Design review of the part built by this model. Coordinates are the model's own, in mm. A direction names the side the tool comes from. Coordinates: 2 decimals unless noted, no trailing zeros. Loops run counter-clockwise (first coordinate to the right, second up) from the corner with the lowest first, then second, coordinate; pieces in that order, holes last.
Q1. Wall thickness on probe 1 along X at (y, z) = (-3.05, -19); probe 2 along Z at (x, y) = (1.5, 2.5); probe 3 along Z at (x, y) = (1.5, 0): over which ranges is each line inside the solid? List them lowest first.
Q2. Add section B-B on x = 3.5. Give the boundary of the cut face in (y, z), and give its area (3 significant figures).
Q3. For P1, Ø2, axis at x = 6.5, y = 0.5, coming from the -Z side; P2, Ø3.5, axis at x = 5, z = -19, coming from the +Y side; P3, Ø5, axis at x = 7.5, z = -13, coming from the +Y side; P4, Ø3, axis at x = 2.5, z = -17.5, coming from the +Y side, all flat-tipped, find the tip position at first contact; note any pin that passes through.
Q4. Draft analysis for pull direction Z (two halves, no side actions). For faces 6 (the face through (0, 2, 0)), 7 (the face through (5, 1, -11.5)), 8 (the face through (5, -4, -3.15)), state which applies: released by +Z, released by -Z, zero draft, split by the parting line, or undercut.
Q5. Machinability: for faces 1 (the face through (2.7, -1, -16.8)), 2 (the face through (5, -4, 3.15)), 3 (the face through (5, 1, 11.5)), 4 (the face through (3.2, -3, -21.4)), 5 (the face through (1, -3, -24)), which of the approach directions +Z, -Z, +X, -X, +Y, -Y give a long, thin tool a straight path to every point of the face, cutting with its end or side? Answer none if there is none.
Q6. Add section C-C on z = 16.5. Give the boundary of the cut face in (x, y), and give its area (3 significant figures).
Q7. Add section A-A on z = -19. Give the boundary of the cut face in (x, y).
Q8. Add section D-D on z = -12.5. Give the boundary of the cut face in (x, y).
```python
from build123d import *

# Parameters (mm, degrees)
SKETCH1_W           = 50
SKETCH1_H           = 10
BOSS_EXTRUDE1_DEPTH = 10
SKETCH3_W           = 10
SKETCH3_H           = 13.5
CUT_EXTRUDE1_DEPTH  = 6
SKETCH4_R           = 3
CUT_EXTRUDE2_DEPTH  = 6
SKETCH5_R           = 3.15
SKETCH5_W           = 6.3
SKETCH5_H           = 7.480912946
CUT_EXTRUDE3_DEPTH  = 28.386127875
CHAMFER1_SIZE       = 2


with BuildPart() as part:
    # Sketch1 → Boss-Extrude1 (new body)
    with BuildSketch(Plane(origin=(0, 0, 0), x_dir=(0, 0, -1), z_dir=(1, 0, 0))):
        Rectangle(SKETCH1_W, SKETCH1_H)
    extrude(amount=BOSS_EXTRUDE1_DEPTH)

    # Sketch3 → Cut-Extrude1 (cut)
    with BuildSketch(Plane(origin=(0, 5, 0), x_dir=(1, 0, 0), z_dir=(0, 1, 0))):
        with Locations((5, -18.25)):
            Rectangle(SKETCH3_W, SKETCH3_H)
        with Locations((5, 18.25)):
            Rectangle(SKETCH3_W, SKETCH3_H)
    extrude(amount=-CUT_EXTRUDE1_DEPTH, mode=Mode.SUBTRACT)

    # Sketch4 → Cut-Extrude2 (cut)
    with BuildSketch(Plane(origin=(0, -1, 0), x_dir=(1, 0, 0), z_dir=(0, 1, 0))):
        with Locations(Location((5, 19, 0), (0, 0, 270))):
            Circle(SKETCH4_R)
        with Locations(Location((5, -19, 0), (0, 0, 270))):
            Circle(SKETCH4_R)
    extrude(amount=-CUT_EXTRUDE2_DEPTH, mode=Mode.SUBTRACT)

    # Sketch5 → Cut-Extrude3 (cut, through all)
    with BuildSketch(Plane(origin=(10, 0, 0), x_dir=(0, 0, -1), z_dir=(1, 0, 0))):
        with Locations((0, -2)):
            Circle(SKETCH5_R)
        with Locations((0, -5.740456473)):
            Rectangle(SKETCH5_W, SKETCH5_H)
    extrude(amount=-CUT_EXTRUDE3_DEPTH, mode=Mode.SUBTRACT)

    # Chamfer1
    chamfer1_edges = [part.edges().sort_by_distance(p)[0] for p in [
        (0, -3, 25),
        (10, -3, 25),
        (5, 5, 11.5),
        (5, 5, -11.5),
        (10, -3, -25),
        (0, -3, -25),
    ]]
    chamfer(chamfer1_edges, length=CHAMFER1_SIZE)


solid = part.part
```
Entries:
1. probe 1: x = 0 to 2, 8 to 10
1. probe 2: z = -11.5 to 11.5
1. probe 3: z = -11.5 to -2.43, 2.43 to 11.5
2. outline: (-5, -25) - (-1, -25) - (-1, -21.6) - (-5, -21.6) - close; (-5, -16.4) - (-1, -16.4) - (-1, -11.5) - (3, -11.5) - (5, -9.5) - (5, 9.5) - (3, 11.5) - (-1, 11.5) - (-1, 16.4) - (-5, 16.4) - (-5, 3.15) - (-2, 3.15) arc R3.15 cw to (-2, -3.15) - (-5, -3.15) - close; (-5, 21.6) - (-1, 21.6) - (-1, 25) - (-5, 25) - close
2. area: 258 mm2
3. P1: stops at z = -11.5
3. P2: passes through
3. P3: stops at y = 4
3. P4: stops at y = -1
4. face 6: zero draft
4. face 7: released by -Z
4. face 8: undercut
5. face 1: -Z, +X, -X, +Y
5. face 2: +X, -X, -Y
5. face 3: +Z, +X, -X, +Y
5. face 4: +Y, -Y
5. face 5: -Z, -X, +Y, -Y
6. outline: (0, -5) - (3.34, -5) - (3.34, -1) - (0, -1) - close; (6.66, -5) - (10, -5) - (10, -1) - (6.66, -1) - close
6. area: 26.7 mm2
7. outline: (0, -5) - (2, -5) - (2, -1) - (0, -1) - close; (8, -5) - (10, -5) - (10, -1) - (8, -1) - close
8. outline: (0, -5) - (10, -5) - (10, -1) - (0, -1) - close
